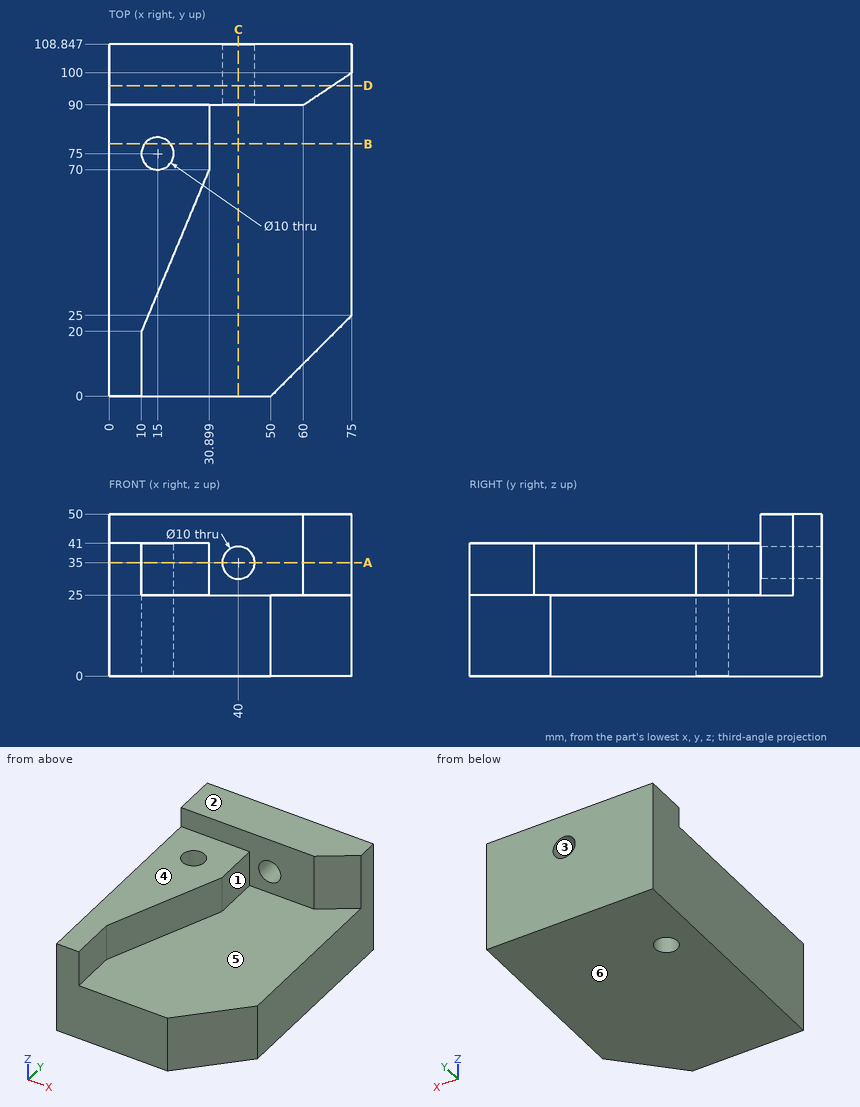
Print and shaded views of the part. All mm, measured from the part's lowest x, y and z. A direction names the side the tool comes from. Round coordinates to 2 decimals unless told otherwise and drop trailing zeros. Write each loop counter-clockwise with the first axis right and the second up, starting at its lowest first coordinate (ties: lowest second). Pieces come first, ordered by that corner, then holes. Notation, with made-up numbers: (-15.75, -13) - (6.25, -13) arc R22 ccw to (6.25, -7) - close; hole circle Ø6 at (67, -39). An arc over 180 degrees is marked (long way). Use CSV: the item, a comma, the result in double quotes. Start each with the question number.
Item 1: Drill centre lines: L1, parallel to X at y = 75, z = 24; L2, parallel to Z at x = 40, y = 99.25; L3, parallel to Z at x = 48, y = 56. Where is each one in solid material? Low to high. Write a range as [from, to].
Item 2: Band-saw the part on D-D (y = 96). Write the cut outline in (x, z).
Item 3: Band-saw the part on B-B (y = 78). Write the cut outline in (x, z), and give its area (3 significant figures).
Item 4: Band-saw the part on A-A (z = 35). Write the cut outline in (x, y).
Item 5: Tool access for the marked faces 4, 5 and 6: list every direction of +Z, -Z, +X, -X, +Y, -Y with a clear straight run to the whole face (end or side of a thin tool).
Item 6: Pin check, flat tips, straight feed: P1, Ø2, axis at y = 82, z = 9.5, coming from the -X side; P2, Ø3, axis at x = 28, z = 43, coming from the -Y side; P3, Ø4, axis at x = 12.5, z = 31, coming from the -Y side (1 decimal); P4, Ø8, axis at y = 7.5, z = 32, coming from the +X side. Stop position of each tip, or through.
Item 7: Two-plate mould, pull along Z, no slides. Class the marked faces 1, 2 and 3: released by +Z, released by -Z, zero draft, split by the parting line, or undercut.
Item 8: Band-saw the part on C-C (x = 40). Write the cut outline in (y, z), and give its area (3 significant figures).
Checked values:
1,L1,"x = [0, 10], [20, 75]"
1,L2,"z = [0, 30], [40, 50]"
1,L3,"z = [0, 25]"
2,outline,"(0, 0) - (75, 0) - (75, 25) - (69, 25) - (69, 50) - (0, 50) - close; hole circle Ø10 at (40, 35)"
3,outline,"(0, 0) - (11, 0) - (11, 41) - (0, 41) - close; (19, 0) - (75, 0) - (75, 25) - (30.9, 25) - (30.9, 41) - (19, 41) - close"
3,area,"2,040 mm²"
4,outline,"(0, 0) - (10, 0) - (10, 20) - (30.9, 70) - (30.9, 90) - (35, 90) - (35, 108.85) - (0, 108.85) - close; (45, 90) - (60, 90) - (75, 100) - (75, 108.85) - (45, 108.85) - close; hole circle Ø10 at (15, 75)"
5,face 4,"+Z, +X, -X, -Y"
5,face 5,"+Z, +X, -Y"
5,face 6,"-Z, +X, -X, +Y, -Y"
6,P1,"stops at x = 0"
6,P2,"stops at y = 90"
6,P3,"stops at y = 21.2"
6,P4,"stops at x = 10"
7,face 1,"zero draft"
7,face 2,"released by +Z"
7,face 3,"undercut"
8,outline,"(0, 0) - (108.85, 0) - (108.85, 30) - (90, 30) - (90, 25) - (0, 25) - close; (90, 40) - (108.85, 40) - (108.85, 50) - (90, 50) - close"
8,area,"3,000 mm²"
